Check sheet for the modelled part. Datum: model origin and axes. Units: mm. Give positions to 0.01 mm unless a question says otherwise; leave off trailing zeros. Order: outer loops, then holes, each group sorted by start corner. A loop starts at its lowest first (then second) coordinate and runs counter-clockwise, first axis right, second up. Notation, with made-up numbers: (-21, -17.5) -> (-9, -17.5) arc R11 ccw to (-9, -6.5) -> close; hole circle Ø3 at (73, 5). An arc over 180 degrees is marked (long way). One line per question, with ' | ' between items. Start each with the question number.
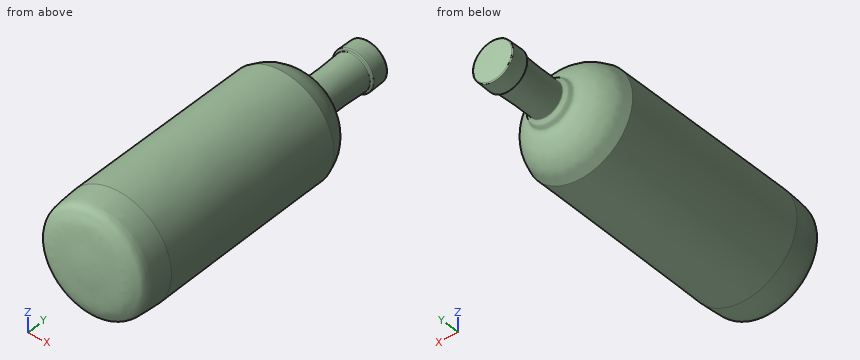
from build123d import *


with BuildPart() as part:
    # Skizze1 → Rotation1 (revolve)
    with BuildSketch(Plane.XY, mode=Mode.PRIVATE) as rotation1_sk:
        with BuildLine():
            Line((118.802046146, 1022.196696021), (176.964475157, 1024.103660907))
            Line((176.964475157, 1024.103660907), (177, 1023.888109373))
            Line((177, 1023.888109373), (177, 0.348553443))
            add(Edge.make_bspline(
                [(177, 0.348553443), (155.865875344, -0.049607015), (134.786920125, 0.63740998), (114, 4), (102.48360535, 5.862946193), (64.153109498, 4.609112023), (44, 16), (37.629076517, 19.600956751), (29.895595043, 21.560449952), (25, 27), (20.402979586, 32.10780046), (18.004259572, 39.201935207), (17, 46), (13.629938224, 68.812725865), (13.666666667, 92), (12, 115)],
                knots=[3.482218919, 3.482218919, 3.482218919, 3.482218919, 4, 4, 4, 5, 5, 5, 6, 6, 6, 7, 7, 7, 8, 8, 8, 8], degree=3))
            Line((12, 115), (14.998694181, 707.741883078))
            add(Edge.make_bspline(
                [(14.998694181, 707.741883078), (20.981370035, 719.493328883), (22.735095514, 733.183933146), (29.26673881, 744.639347794), (35.739688358, 755.99182338), (44.18359103, 766.291093776), (53.490993869, 775.464426331), (62.465440762, 784.309599068), (73.152898477, 791.286271073), (83.657055799, 798.246188942), (90.620513231, 802.860085166), (99.269721474, 804.807300601), (105.743529772, 810.086276249), (109.332407544, 813.012775998), (110.025107715, 818.350781682), (112.830398448, 822.035179645), (116.117568409, 826.352465608), (123.574773092, 828.539604738), (123.91716187, 833.955065417), (126.673177858, 877.546144248), (122.550765948, 921.300609512), (121.867567987, 964.97338156)],
                knots=[0, 0, 0, 0, 1, 1, 1, 2, 2, 2, 3, 3, 3, 4, 4, 4, 5, 5, 5, 6, 6, 6, 7, 7, 7, 7], degree=3))
            ThreePointArc((121.867567987, 964.97338156), (121.292270479, 966.686317901), (119.837491405, 967.758108914))
            Line((119.837491405, 967.758108914), (116.86842359, 968.771936948))
            ThreePointArc((116.86842359, 968.771936948), (115.378415373, 969.893093626), (114.838602637, 971.677951881))
            Line((114.838602637, 971.677951881), (115.901101463, 1019.265272556))
            ThreePointArc((115.901101463, 1019.265272556), (116.767977156, 1021.308513129), (118.802046146, 1022.196696021))
        make_face()
    revolve(rotation1_sk.sketch.rotate(Axis((177, 1120.97176066, 0), (0, -1, 0)), 270), axis=Axis((177, 1120.97176066, 0), (0, -1, 0)))  # turned: the seam where the file's is


solid = part.part
1. Cross-section at A-A on y = 148. Record the boundary of the cut face in (x, z), and give its area (3 significant figures).
2. Cross-section at B-B on y = 341. Record the boundary of the cut face in (x, z), and give its area (3 significant figures).
3. Scan lines: probe 1 along Z at (x, y) = (100, 416); probe 2 along Y at (x, z) = (307.5, 63); probe 3 along Y at (x, z) = (187, 77.5). Record each from-to range of solid material in increasing order.
4. Go/stop test with flat-tipped pins: pin 1 (12 mm diameter, centred on y = 270.5, z = -100.5, fed in from -X); pin 2 (1.5 mm diameter, centred on x = 80.5, y = 210.5, fed in from -Z); pin 3 (5 mm diameter, centred on x = 132, z = -107.5, fed in from -Y). Record where each tip stops, or that it passes through.
Response values:
1) outline: circle Ø329.67 at (177, 0) | area: 85,400 mm²
2) outline: circle Ø327.71 at (177, 0) | area: 84,300 mm²
3) probe 1: z = -144.21 to 144.21 | probe 2: y = 21.75 to 749.33 | probe 3: y = 5.19 to 805.78
4) pin 1: stops at x = 42.7 | pin 2: stops at z = -133.78 | pin 3: stops at y = 9.33
